The figure shows three views and two pictorial views of one solid part (mm, origin at its lowest corner). Answer the questions. A direction names the side the tool comes from. Coordinates: 2 decimals unless noted, no trailing zeros. Loops run counter-clockwise (first coordinate to the right, second up) from the corner with the lowest first, then second, coordinate; pieces in that order, holes last.
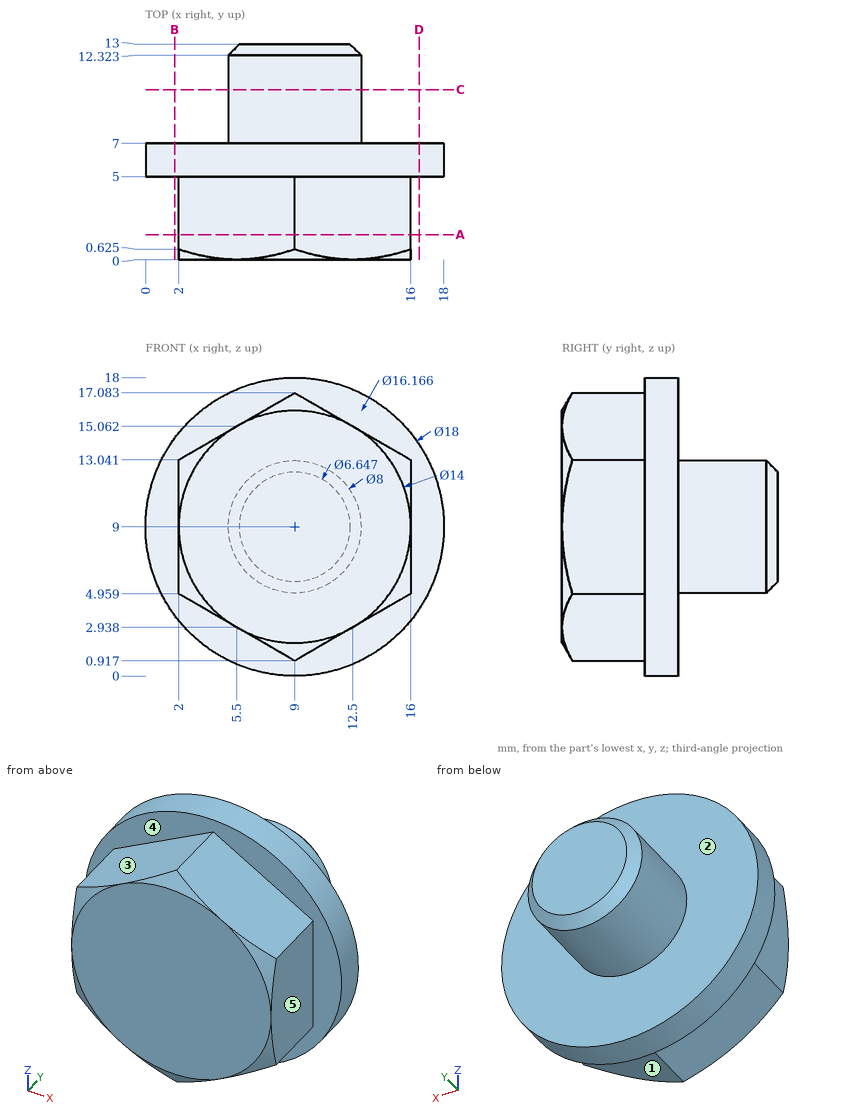
Q1. A cutting plane is placed at B-B (x = 1.75). Give the vertices of the cut face in (y, z).
Findings below:
outline: (5, 3.67) - (7, 3.67) - (7, 14.33) - (5, 14.33) - close
Q2. A cutting plane is placed at D-D (x = 16.5). Give the vertices of the cut face in (y, z) (1 decimal), then the cut area to 3 significant figures.
Findings below:
outline: (5, 4) - (7, 4) - (7, 14) - (5, 14) - close
area: 19.9 mm2
Q3. Which of the six approach directions +Z, -Z, +X, -X, +Y, -Y give full straight-line access (tool end or side, diameter ignored) to the marked faces 1, 2, 3, 4 and 5?
Findings below:
face 1: -Z, +X, -Y
face 2: +Y
face 3: +Z, -X, -Y
face 4: -Y
face 5: +Z, -Z, +X, -Y
Q4. Straight lines are drawn through the part: probe 1 along Y at (x, z) = (11.5, 15); probe 2 along Y at (x, z) = (6.25, 1); probe 3 along X at (y, z) = (4, 9.25). For each, find the intervals that lie inside material, in ascending order.
Findings below:
probe 1: y = 0 to 7
probe 2: y = 5 to 7
probe 3: x = 2 to 16
Q5. Flat-ended cylindrical pins translate along their axes: pin 1 Ø1.5 at (y, z) = (1.5, 9) entering from -X; pin 2 Ø2.5 at (y, z) = (2.5, 9.5) entering from +X; pin 3 Ø4 at (x, y) = (12, 4.5) entering from -Z. Find the tip coordinate at first contact, or state that the pin passes through.
Findings below:
pin 1: stops at x = 2
pin 2: stops at x = 16
pin 3: stops at z = 0.06
Q6. A cutting plane is placed at A-A (y = 1.5). Give the vertices of the cut face in (x, z), then the cut area to 3 significant figures.
Findings below:
outline: (2, 4.96) - (9, 0.92) - (16, 4.96) - (16, 13.04) - (9, 17.08) - (2, 13.04) - close
area: 170 mm2
Q7. A cutting plane is placed at C-C (y = 10.25). Give the vertices of the cut face in (x, z).
Findings below:
outline: circle Ø8 at (9, 9)
